For this review, take the finished solid that the model builds, in its own axes (mm). A direction names the side the tool comes from. Round coordinates to 2 decimals unless told otherwise and drop trailing zeros. Order: outer loops, then holes, each group sorted by start corner. A loop starts at its lowest first (then second) coordinate and runs counter-clockwise, first axis right, second up. Notation, with made-up numbers: M 46,42 L 102,42 A34 ccw 102,79 Z; hole C -34,85.5 d6. An arc over 180 degrees is marked long. Put each result on its own line as item: value.
from build123d import *

# Parameters (mm, degrees)
PAD_DEPTH       = 27
POCKET_DEPTH    = 8
SKETCH002_R     = 3.5
POCKET001_DEPTH = 5
POCKET002_DEPTH = 17
SKETCH004_R     = 1
POCKET003_DEPTH = 11
SKETCH005_W     = 12
SKETCH005_H     = 4
POCKET004_DEPTH = 7
POCKET005_DEPTH = 1.3
POCKET006_DEPTH = 2
SKETCH011_R     = 0.75
POCKET008_DEPTH = 12
POCKET009_DEPTH = 5


with BuildPart() as part:
    # Sketch → Pad (new body)
    with BuildSketch(Plane.XY):
        with BuildLine():
            Line((-9, 47.5), (9, 47.5))
            ThreePointArc((17, 39.5), (14.656854, 45.156854), (9, 47.5))
            Line((17, 39.5), (17, -38.5))
            ThreePointArc((9, -46.5), (14.656854, -44.156854), (17, -38.5))
            Line((-9, -46.5), (9, -46.5))
            ThreePointArc((-17, -38.5), (-14.656854, -44.156854), (-9, -46.5))
            Line((-17, 39.5), (-17, -38.5))
            ThreePointArc((-9, 47.5), (-14.656854, 45.156854), (-17, 39.5))
        make_face()
    extrude(amount=PAD_DEPTH)

    # Sketch001 (on Face10 of Pad) → Pocket (cut)
    with BuildSketch(Plane.XY.offset(27)):
        with BuildLine():
            Line((-9, 45.5), (9, 45.5))
            ThreePointArc((15, 39.5), (13.242641, 43.742641), (9, 45.5))
            Line((15, 39.5), (15, -38.5))
            ThreePointArc((9, -44.5), (13.242641, -42.742641), (15, -38.5))
            Line((-9, -44.5), (9, -44.5))
            ThreePointArc((-15, -38.5), (-13.242641, -42.742641), (-9, -44.5))
            Line((-15, 39.5), (-15, -38.5))
            ThreePointArc((-9, 45.5), (-13.242641, 43.742641), (-15, 39.5))
        make_face()
    extrude(amount=-POCKET_DEPTH, mode=Mode.SUBTRACT)

    # Sketch002 (on Face2 of Pocket) → Pocket001 (cut)
    with BuildSketch(Plane(origin=(0, 47.5, 0), x_dir=(-1, 0, 0), z_dir=(0, 1, 0))):
        with Locations((-1.9, 21)):
            Circle(SKETCH002_R)
    extrude(amount=-POCKET001_DEPTH, mode=Mode.SUBTRACT)

    # Sketch003 (on Face20 of Pocket001) → Pocket002 (cut)
    with BuildSketch(Plane.XY.offset(19)):
        with BuildLine():
            ThreePointArc((8, 39.5), (8.709006, 37.972475), (10.333333, 37.527973))
            ThreePointArc((15, 33.58392), (13.581989, 36.638971), (10.333333, 37.527973))
            Line((15, -35), (15, 33.58392))
            ThreePointArc((12, -38), (14.12132, -37.12132), (15, -35))
            ThreePointArc((12, -38), (10.725245, -38.709431), (10.65629, -40.166667))
            ThreePointArc((7.968871, -44.5), (10.518381, -43.081139), (10.65629, -40.166667))
            Line((7.968871, -44.5), (-9, -44.5))
            ThreePointArc((-15, -38.5), (-13.242641, -42.742641), (-9, -44.5))
            Line((-15, -38.5), (-15, 33.58392))
            ThreePointArc((-10.333333, 37.527973), (-13.581989, 36.638971), (-15, 33.58392))
            ThreePointArc((-10.333333, 37.527973), (-8.46929, 38.212783), (-8.114382, 40.166667))
            ThreePointArc((-4.343146, 45.5), (-7.609132, 43.809401), (-8.114382, 40.166667))
            Line((6.5, 45.5), (-4.343146, 45.5))
            ThreePointArc((8, 44), (7.56066, 45.06066), (6.5, 45.5))
            Line((8, 39.5), (8, 44))
        make_face()
    extrude(amount=-POCKET002_DEPTH, mode=Mode.SUBTRACT)

    # Sketch004 (on Face15 of Pocket002) → Pocket003 (cut)
    with BuildSketch(Plane.XY.offset(19)):
        with Locations((-10, 39.5)):
            Circle(SKETCH004_R)
        with Locations((10, 39.5)):
            Circle(SKETCH004_R)
        with Locations((12, -39.5)):
            Circle(SKETCH004_R)
    extrude(amount=-POCKET003_DEPTH, mode=Mode.SUBTRACT)

    # Sketch005 (on Face5 of Pocket003) → Pocket004 (cut)
    with BuildSketch(Plane.XY.offset(27)):
        with Locations((4, -44.5)):
            Rectangle(SKETCH005_W, SKETCH005_H)
    extrude(amount=-POCKET004_DEPTH, mode=Mode.SUBTRACT)

    # Sketch007 (on Face26 of Pocket004) → Pocket005 (cut)
    with BuildSketch(Plane.XY.offset(2)):
        with BuildLine():
            ThreePointArc((8, 32.5), (0, 40.5), (-8, 32.5))
            Line((-8, 32.5), (-8, -32.5))
            ThreePointArc((-8, -32.5), (0, -40.5), (8, -32.5))
            Line((8, 32.5), (8, -32.5))
        make_face()
        with BuildLine():
            ThreePointArc((15, 31), (12, 34), (9, 31))
            Line((9, 31), (9, 6))
            ThreePointArc((9, 6), (12, 3), (15, 6))
            Line((15, 31), (15, 6))
        make_face()
    extrude(amount=-POCKET005_DEPTH, mode=Mode.SUBTRACT)

    # Sketch008 (on Face5 of Pocket005) → Pocket006 (cut)
    with BuildSketch(Plane.XY.offset(27)):
        with BuildLine():
            Line((-9, 46.5), (9, 46.5))
            ThreePointArc((16, 39.5), (13.949747, 44.449747), (9, 46.5))
            Line((16, 39.5), (16, -38.5))
            ThreePointArc((9, -45.5), (13.949747, -43.449747), (16, -38.5))
            Line((-9, -45.5), (9, -45.5))
            ThreePointArc((-16, -38.5), (-13.949747, -43.449747), (-9, -45.5))
            Line((-16, 39.5), (-16, -38.5))
            ThreePointArc((-9, 46.5), (-13.949747, 44.449747), (-16, 39.5))
        make_face()
    extrude(amount=-POCKET006_DEPTH, mode=Mode.SUBTRACT)

    # Sketch011 (on Face24 of Pocket006) → Pocket008 (cut)
    with BuildSketch(Plane.XY.offset(25)):
        with Locations((-10, 44.5)):
            Circle(SKETCH011_R)
        with Locations((12, -43.5)):
            Circle(SKETCH011_R)
    extrude(amount=-POCKET008_DEPTH, mode=Mode.SUBTRACT)

    # Sketch012 (on Face11 of Pocket008) → Pocket009 (cut)
    with BuildSketch(Plane.XZ.offset(46.5)):
        with BuildLine():
            Line((0, 0), (0, 10))
            ThreePointArc((0, 10), (-1.171573, 12.828427), (-4, 14))
            Line((-9, 14), (-4, 14))
            ThreePointArc((-9, 14), (-11.828427, 12.828427), (-13, 10))
            Line((-13, 10), (-13, 0))
            Line((-13, 0), (0, 0))
        make_face()
    extrude(amount=-POCKET009_DEPTH, mode=Mode.SUBTRACT)


solid = part.part
(1) For faces 1 (the face through (-11.797, -44.761, 12.859)), 2 (the face through (8, 42, 11)), 3 (the face through (14.594, -44.219, 13.311)), list the 3-axis set-ups (+Z, -Z, +X, -X, +Y, -Y) from which the entire face can be reached by the end or side of a thin tool; tool diameter is ignored.
A:
face 1: -Z, -Y
face 2: +Z
face 3: +Z, -Z, +X, -Y
(2) Add section B-B on y = -8. Give the boundary of the cut face in (x, z).
A:
outline: M -17,0 L 17,0 L 17,27 L 16,27 L 16,25 L 15,25 L 15,2 L 8,2 L 8,0.7 L -8,0.7 L -8,2 L -15,2 L -15,25 L -16,25 L -16,27 L -17,27 Z
(3) To check wall thickness, follow L1, parallel to X at y = 17, z = 22; L2, parallel to Y at x = 1, z = 9.5; L3, parallel to Y at x = -10, z = 16.1. State the ranges of each line that lie inside material, in increasing order.
A:
L1: x = -17 to -15, 15 to 17
L2: y = -46.5 to -44.5, 45.5 to 47.5
L3: y = -46.44 to -44.42, 37.5 to 38.5, 40.5 to 43.75, 45.25 to 47.44
(4) Draft analysis for pull direction Y (two halves, no side actions). For faces 4 (the face through (0, 47.5, 13)), 5 (the face through (16, 1, 26)), 6 (the face through (-1.141, -45.514, 12.797)), state which applies: released by +Y, released by -Y, zero draft, split by the parting line, or undercut.
A:
face 4: released by +Y
face 5: undercut
face 6: zero draft
(5) Add section D-D on z = 15.75. Give the boundary of the cut face in (x, y).
A:
outline: M -17,-38.5 A8 ccw -9,-46.5 L 9,-46.5 A8 ccw 17,-38.5 L 17,39.5 A8 ccw 9,47.5 L -9,47.5 A8 ccw -17,39.5 Z; hole M -15,-38.5 A6 ccw -9,-44.5 L 7.97,-44.5 A3 ccw 10.66,-40.17 A1.5 cw 12,-38 A3 ccw 15,-35 L 15,33.58 A4 ccw 10.33,37.53 A2 cw 8,39.5 L 8,44 A1.5 ccw 6.5,45.5 L -4.34,45.5 A4 ccw -8.11,40.17 A2 cw -10.33,37.53 A4 ccw -15,33.58 Z; hole C -10,39.5 d2; hole C -10,44.5 d1.5; hole C 10,39.5 d2; hole C 12,-39.5 d2; hole C 12,-43.5 d1.5
(6) Add section A-A on z = 21. Give the boundary of the cut face in (x, y).
A:
outline: M -17,-38.5 A8 ccw -9,-46.5 L -2,-46.5 L -2,-44.5 L -9,-44.5 A6 cw -15,-38.5 L -15,39.5 A6 cw -9,45.5 L -1.6,45.5 L -1.6,47.5 L -9,47.5 A8 ccw -17,39.5 Z; M 5.4,45.5 L 9,45.5 A6 cw 15,39.5 L 15,-38.5 A6 cw 12.7,-43.23 A0.75 cw 11.43,-43.99 A6 cw 10,-44.42 L 10,-46.44 A8 ccw 17,-38.5 L 17,39.5 A8 ccw 9,47.5 L 5.4,47.5 Z
(7) Add section C-C on x = -5.5. Give the boundary of the cut face in (y, z), then the cut area to 3 significant figures.
A:
outline: M -46.5,14 L -44.5,14 L -44.5,25 L -45.5,25 L -45.5,27 L -46.5,27 Z; M -41.5,0 L 47.5,0 L 47.5,27 L 46.5,27 L 46.5,25 L 45.5,25 L 45.5,19 L 45.33,19 L 45.33,2 L 38.31,2 L 38.31,0.7 L -38.31,0.7 L -38.31,2 L -41.5,2 Z
area: 153 mm2
(8) Insertion check: pin 1 Ø2 at (x, y) = (-5.5, -46) entering from -Z; pin 2 Ø3 at (x, y) = (12, 33.5) entering from +Z; pin 3 Ø1.5 at (x, y) = (-7, 2.5) entering from -Z; pin 4 Ø1 at (x, z) = (11, 5) entering from +Y. Each pin has a flat end and moves straight along its axis. Give the tip position at first contact, or say it passes through.
A:
pin 1: stops at z = 14
pin 2: stops at z = 2
pin 3: stops at z = 0
pin 4: stops at y = 47.36
